Verification items for this drawing (mm, ordinates from the low corner). A direction names the side the tool comes from. Give positions to 0.01 mm unless a question says otherwise; leave off trailing zeros. Order: outer loops, then holes, each group sorted by start corner. A loop starts at its lowest first (then second) coordinate and runs counter-clockwise, first axis right, second up. Notation, with made-up numbers: (27, -11) -> (39, -11) arc R10 ccw to (39, -7) -> close; hole circle Ø7 at (89.5, -13.5). An arc over 180 degrees is marked (long way). One line per question, with ' | ' between items.
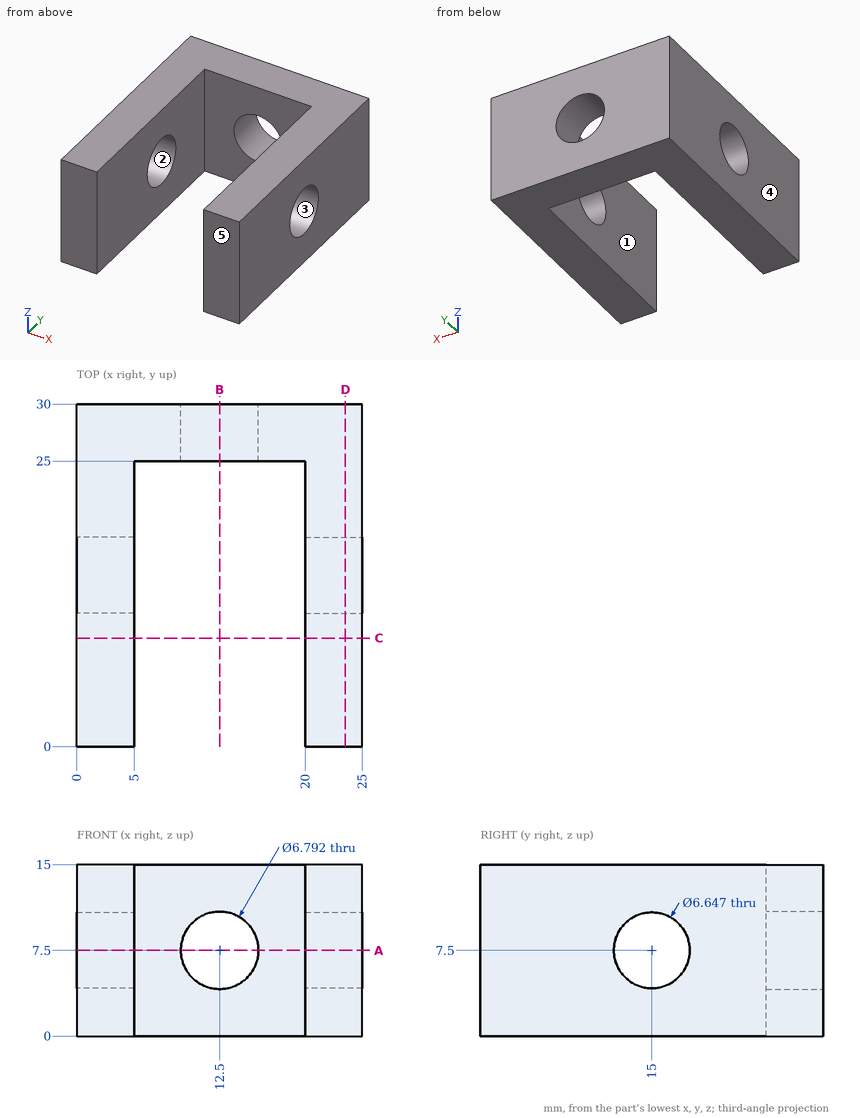
Q1. Section check C-C (y = 9.5). Enter the section's corners in (x, z).
Result sheet:
outline: (0, 0) -> (5, 0) -> (5, 15) -> (0, 15) -> close; (20, 0) -> (25, 0) -> (25, 15) -> (20, 15) -> close
Q2. Section check B-B (x = 12.5). Enter the section's corners in (y, z), and give its area (3 significant figures).
Result sheet:
outline: (25, 0) -> (30, 0) -> (30, 4.1) -> (25, 4.1) -> close; (25, 10.9) -> (30, 10.9) -> (30, 15) -> (25, 15) -> close | area: 41.0 mm2
Q3. Thickness scan on line 1 (X direction, y = 14, z = 12); line 2 (Z direction, x = 3.25, y = 15); line 3 (Z direction, x = 12.5, y = 28.5). Record the ranges inside material, lowest first.
Result sheet:
line 1: x = 0 to 5, 20 to 25 | line 2: z = 0 to 4.18, 10.82 to 15 | line 3: z = 0 to 4.1, 10.9 to 15
Q4. Section check D-D (x = 23.5). Enter the section's corners in (y, z), and give its area (3 significant figures).
Result sheet:
outline: (0, 0) -> (30, 0) -> (30, 15) -> (0, 15) -> close; hole circle Ø6.65 at (15, 7.5) | area: 415 mm2
Q5. Mould release check, pull along Y, two halves, no side actions. Record for the marked faces 3, 4 and 5: pulls with the +Y half, pulls with the -Y half, needs draft (parallel to the pull), parting line crosses it, or undercut.
Result sheet:
face 3: undercut | face 4: needs draft | face 5: pulls with the -Y half
Q6. Access from +Z, -Z, +X, -X, +Y, -Y to the whole of each face (thin tool, end or side, straight path). Record for the marked faces 1 and 2.
Result sheet:
face 1: +Z, -Z, -Y | face 2: +X, -X
Q7. Section check A-A (z = 7.5). Enter the section's corners in (x, y).
Result sheet:
outline: (0, 0) -> (5, 0) -> (5, 11.68) -> (0, 11.68) -> close; (0, 18.32) -> (5, 18.32) -> (5, 25) -> (9.1, 25) -> (9.1, 30) -> (0, 30) -> close; (15.9, 25) -> (20, 25) -> (20, 18.32) -> (25, 18.32) -> (25, 30) -> (15.9, 30) -> close; (20, 0) -> (25, 0) -> (25, 11.68) -> (20, 11.68) -> close
